```python
from build123d import *

# Parameters (mm, degrees)
SKETCH_1_R            = 8
EXTRUDE_1_DEPTH       = 21
HOLE_WIZARD_M5_1_D    = 4.2
HOLE_WIZARD_5_0_5_1_D = 5


with BuildPart() as part:
    # 草图1 → 凸台-拉伸1 (new body)
    with BuildSketch(Plane.XY):
        Polygon((8, 0), (-8, 0), (-8, 1), (-13, 6), (-25, 6), (-25, 38.5), (25, 38.5), (25, 6), (13, 6), (8, 1), align=None)
        with Locations(Location((0, 19.5, 0), (0, 0, 180))):
            Circle(SKETCH_1_R, mode=Mode.SUBTRACT)
    extrude(amount=EXTRUDE_1_DEPTH)

    # M5 螺纹孔1 (through all)
    with Locations(Plane.XY.offset(21)):
        with Locations((-21.2, 19.5), (21.2, 19.5)):
            Hole(HOLE_WIZARD_M5_1_D / 2)

    # Ø5.0 (5) 直径孔1 (through all)
    with Locations(Plane(origin=(0, 38.5, 0), x_dir=(1, 0, 0), z_dir=(0, 1, 0))):
        with Locations((-18, -16), (18, -16)):
            Hole(HOLE_WIZARD_5_0_5_1_D / 2)


solid = part.part
```
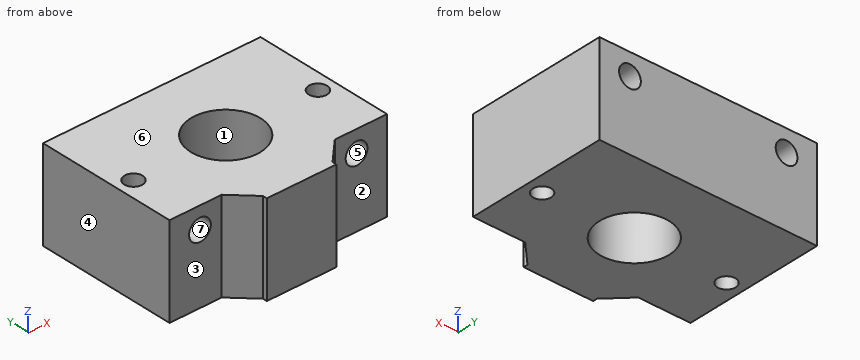
Geometry: final body of the model. Coordinates: model frame, mm. Face numbers are marked on the shaded views. A direction names the side the tool comes from. Round coordinates to 2 decimals unless told otherwise and drop trailing zeros. Order: outer loops, then holes, each group sorted by start corner. A loop starts at its lowest first (then second) coordinate and runs counter-clockwise, first axis right, second up. Notation, with made-up numbers: (62.25, 0.25) -> (106.25, 0.25) arc R7 cw to (106.25, 5.25) -> close; hole circle Ø4 at (-16, 53). An arc over 180 degrees is marked (long way). Use one line per item in the form item = value.
(1) Section B-B on y = 15. Return loops of the section in (x, z), and give its area (3 significant figures).
Results list:
outline = (-25, 0) -> (-6.61, 0) -> (-6.61, 21) -> (-25, 21) -> close; (6.61, 0) -> (25, 0) -> (25, 21) -> (6.61, 21) -> close; hole circle Ø5 at (-18, 16); hole circle Ø5 at (18, 16)
area = 733 mm^2
(2) Access query for the marked faces 1, 2 and 3. Directions: +Z, -Z, +X, -X, +Y, -Y. A direction counts if a zero-diameter tool reaches every point of the face in a straight line with its end or side. Return the directions, or none.
Results list:
face_1 = +Z, -Z
face_2 = +Z, -Z, +X, -Y
face_3 = +Z, -Z, -X, -Y
(3) First-contact query: pin 1 Ø0.5 at (y, z) = (0.5, 12) entering from -X; pin 2 Ø6 at (x, z) = (20.5, 8.5) entering from -Y. Flat tips, straight axial feed; report the tip coordinate or a pass-through.
Results list:
pin_1 = -8
pin_2 = 6
(4) Ray query, probe 1 along Z at (x, y) = (-18, 22.5); probe 2 along Y at (x, z) = (-21, 3.5); probe 3 along X at (y, z) = (8.5, 14). Return the intervals inside material, ascending. Write a range as [from, to].
Results list:
probe_1 = [0, 13.5], [18.5, 21]
probe_2 = [6, 17.41], [21.59, 38.5]
probe_3 = [-25, -19.5], [-16.5, 16.5], [19.5, 25]
(5) Section C-C on z = 12.25. Return loops of the section in (x, y), and give its area (3 significant figures).
Results list:
outline = (-25, 6) -> (-13, 6) -> (-8, 1) -> (-8, 0) -> (8, 0) -> (8, 1) -> (13, 6) -> (25, 6) -> (25, 38.5) -> (-25, 38.5) -> close; hole circle Ø4.2 at (-21.2, 19.5); hole circle Ø16 at (0, 19.5); hole circle Ø4.2 at (21.2, 19.5)
area = 1,520 mm^2
(6) Section A-A on x = -21.2. Return loops of the section in (y, z).
Results list:
outline = (6, 0) -> (17.4, 0) -> (17.4, 21) -> (6, 21) -> close; (21.6, 0) -> (38.5, 0) -> (38.5, 21) -> (21.6, 21) -> close
(7) Section D-D on y = 31. Return loops of the section in (x, z), and give its area (3 significant figures).
Results list:
outline = (-25, 0) -> (25, 0) -> (25, 21) -> (-25, 21) -> close; hole circle Ø5 at (-18, 16); hole circle Ø5 at (18, 16)
area = 1,010 mm^2
(8) Draft query along Z for the marked faces 4, 5, 6 and 7. Return one class per face: pulls with the +Z half, pulls with the -Z half, needs draft (parallel to the pull), parting line crosses it, or undercut.
Results list:
face_4 = needs draft
face_5 = undercut
face_6 = pulls with the +Z half
face_7 = undercut
